```python
from build123d import *

# Parameters (mm, degrees)
SKETCH1_W            = 176
SKETCH1_H            = 90
SKETCH1_W_2          = 161
SKETCH1_H_2          = 80.5
BOSS_EXTRUDE1_DEPTH  = 5
M4_CLEARANCE_HOLE1_D = 4.5
BOSS_EXTRUDE2_DEPTH  = 90
BOSS_EXTRUDE11_DEPTH = 176
CUT_EXTRUDE1_DEPTH   = 20
BOSS_EXTRUDE12_DEPTH = 20
BOSS_EXTRUDE13_DEPTH = 5


with BuildPart() as part:
    # Sketch1 → Boss-Extrude1 (new body)
    with BuildSketch(Plane.XY):
        Rectangle(SKETCH1_W, SKETCH1_H)
        Rectangle(SKETCH1_W_2, SKETCH1_H_2, mode=Mode.SUBTRACT)
    extrude(amount=BOSS_EXTRUDE1_DEPTH)

    # M4 Clearance Hole1 (through all)
    with Locations(Plane.XY.offset(5)):
        with Locations((84, 40), (-84, -40), (-84, 40), (84, -40)):
            Hole(M4_CLEARANCE_HOLE1_D / 2)

    # Sketch7 → Boss-Extrude2 (add)
    with BuildSketch(Plane(origin=(0, 45, 0), x_dir=(1, 0, 0), z_dir=(0, 1, 0))):
        Polygon((-82.5, -5), (-88, -25.886602241), (-86, -25.886602241), (-80.5, -5), align=None)
        Polygon((80.5, -5), (60.5, -30.264322131), (62.5, -30.264322131), (82.5, -5), align=None)
    extrude(amount=-BOSS_EXTRUDE2_DEPTH)


with BuildPart() as body_2:
    # Sketch8 → Boss-Extrude11 (new body)
    with BuildSketch(Plane(origin=(88, 0, 0), x_dir=(0, 0, -1), z_dir=(1, 0, 0))):
        Polygon((-5, 40.25), (-30.264322131, 22.5), (-30.264322131, 25), (-5, 42.75), align=None)
    extrude(amount=-BOSS_EXTRUDE11_DEPTH)


with BuildPart() as body_3:
    # Mirror2: mirrored copy
    add(body_2.part.mirror(Plane.ZX))


with BuildPart() as body_2_1:
    add(body_2.part)

    # Combine2: union body 3, part
    add(body_3.part)
    add(part.part)

    # Sketch9 → Cut-Extrude1 (cut)
    with BuildSketch(Plane.XY.offset(5)):
        with BuildLine():
            Line((84, 37.75), (84, 35))
            ThreePointArc((84, 35), (86.236067977, 35.527864045), (88, 37))
            Line((88, 37), (88, 40.25))
            Line((88, 40.25), (86.236067977, 40.25))
            ThreePointArc((86.236067977, 40.25), (85.677050983, 38.5), (84, 37.75))
        make_face()
        with BuildLine():
            ThreePointArc((89, 40), (84, 45), (79, 40))
            Line((79, 40), (84, 40))
            Line((84, 40), (84, 37.75))
            ThreePointArc((84, 37.75), (85.677050983, 38.5), (86.236067977, 40.25))
            Line((86.236067977, 40.25), (88, 40.25))
            Line((88, 40.25), (88, 37))
            ThreePointArc((88, 37), (88.74341649, 38.41886117), (89, 40))
        make_face()
        with BuildLine():
            ThreePointArc((79, 40), (79.968871126, 37.041960108), (82.5, 35.230303993))
            Line((82.5, 35.230303993), (82.5, 38.322949017))
            ThreePointArc((82.5, 38.322949017), (83.197150298, 37.898112192), (84, 37.75))
            Line((84, 37.75), (84, 40))
            Line((84, 40), (79, 40))
        make_face()
        with BuildLine():
            Line((82.5, 38.322949017), (82.5, 35.230303993))
            ThreePointArc((82.5, 35.230303993), (83.241211504, 35.057911371), (84, 35))
            Line((84, 35), (84, 37.75))
            ThreePointArc((84, 37.75), (83.197150298, 37.898112192), (82.5, 38.322949017))
        make_face()
    extrude(amount=CUT_EXTRUDE1_DEPTH, mode=Mode.SUBTRACT)

    # Sketch10 → Boss-Extrude12 (add)
    with BuildSketch(Plane.XY.offset(5)):
        with BuildLine():
            Line((88, 35.527864045), (88, 37))
            ThreePointArc((88, 37), (85.531488162, 35.240321018), (82.5, 35.230303993))
            Line((82.5, 35.230303993), (82.5, 34.190524981))
            ThreePointArc((82.5, 34.190524981), (85.417610293, 34.169872981), (88, 35.527864045))
        make_face()
        with BuildLine():
            Line((82.5, 34.190524981), (82.5, 35.230303993))
            ThreePointArc((82.5, 35.230303993), (81.429126737, 35.711572472), (80.5, 36.429285786))
            ThreePointArc((80.5, 36.429285786), (79.343242015, 38.179394313), (79.006253911, 40.25))
            ThreePointArc((79.006253911, 40.25), (79.24786884, 41.554750602), (79.824176728, 42.75))
            Line((79.824176728, 42.75), (78.667317748, 42.75))
            ThreePointArc((78.667317748, 42.75), (78.523911995, 37.547968157), (82.5, 34.190524981))
        make_face()
        with BuildLine():
            ThreePointArc((79.824176728, 42.75), (80.140212612, 43.178370859), (80.5, 43.570714214))
            Line((80.5, 43.570714214), (80.5, 44.873397172))
            ThreePointArc((80.5, 44.873397172), (79.457833906, 43.920296822), (78.667317748, 42.75))
            Line((78.667317748, 42.75), (79.824176728, 42.75))
        make_face()
    extrude(amount=BOSS_EXTRUDE12_DEPTH)

    # Sketch11 → Boss-Extrude13 (add)
    with BuildSketch(Plane.XY.offset(5)):
        with BuildLine():
            Line((80.5, 35.126602828), (80.5, 40.25))
            Line((80.5, 40.25), (78.005210596, 40.25))
            ThreePointArc((78.005210596, 40.25), (78.605553216, 37.373225572), (80.5, 35.126602828))
        make_face()
    extrude(amount=-BOSS_EXTRUDE13_DEPTH)


solid = body_2_1.part
```
For this review, take the finished solid that the model builds, in its own axes (mm). A direction names the side the tool comes from. Give positions to 0.01 mm unless a question says otherwise; leave off trailing zeros. Loops run counter-clockwise (first coordinate to the right, second up) from the corner with the lowest first, then second, coordinate; pieces in that order, holes last. Notation, with made-up numbers: M 89,75.25 L 94,75.25 A20 ccw 94,103.25 Z; hole C 64.5,38 d6. An arc over 180 degrees is marked long. One line per item, written item: value. Start each with the question number.
Q1. Draft analysis for pull direction Y (two halves, no side actions). For faces 1 (the face through (0, 44, 0)), 2 (the face through (78.262, -31.779, 20.616)), 3 (the face through (72.36, -1.09, 17.81)), state which applies: released by +Y, released by -Y, zero draft, split by the parting line, or undercut.
Q2. Add section D-D (y = -33). Give the boundary of the cut face in (x, z), and give its area (3 significant figures).
Q3. Clearance check with flat-ended pins moving along their axes: pin 1 Ø1 at (x, z) = (-43, 12) entering from +Y; pin 2 Ø5 at (x, y) = (-84, 40) entering from +Z; pin 3 Ø8 at (y, z) = (-24.5, 15) entering from +X; pin 4 Ø3 at (x, y) = (-83, 40) entering from -Z. State where each tip first meets the part, or that it passes through.
Q4. Machinability: for faces 4 (the face through (-80.5, -1, 2)), 5 (the face through (81, 40, 5)), 6 (the face through (-83.9, -38.3, 17.91)), which of the approach directions +Z, -Z, +X, -X, +Y, -Y give a long, thin tool a straight path to every point of the face, cutting with its end or side? Answer none if there is none.
Q5. Add section A-A (y = -4). Give the boundary of the cut face in (x, z), and give its area (3 significant figures).
Q6. For L1, parallel to X at y = -40, z = 3; L2, parallel to Y at x = -53, z = 2.5; L3, parallel to Y at x = -34, z = 28.5, list the stretches that pass through material, from the lowest coordinate up.
Q7. Add section B-B (x = -1.5). Give the boundary of the cut face in (y, z).
Q8. Add section C-C (z = 21.5). Count the separate pieces of the cut face and the enclosed holes in it, and give its area (3 significant figures).
Reply:
1. face 1: zero draft
1. face 2: released by -Y
1. face 3: undercut
2. outline: M -88,0 L -80.5,0 L -80.5,5 L -83.22,15.32 L 72.33,15.32 L 80.5,5 L 80.5,0 L 88,0 L 88,5 L 82.5,5 L 74.33,15.32 L 88,15.32 L 88,18.88 L 71.51,18.88 L 62.5,30.26 L 60.5,30.26 L 69.51,18.88 L -84.15,18.88 L -86,25.89 L -88,25.89 L -86.15,18.88 L -88,18.88 L -88,15.32 L -85.22,15.32 L -82.5,5 L -88,5 Z
2. area: 779 mm²
3. pin 1: y = 38.18
3. pin 2: z = 25.89
3. pin 3: x = 77.75
3. pin 4: z = 0
4. face 4: -Z
4. face 5: +Z
4. face 6: +Z, -Y
5. outline: M -88,0 L -80.5,0 L -80.5,5 L -86,25.89 L -88,25.89 L -82.5,5 L -88,5 Z; M 60.5,30.26 L 80.5,5 L 80.5,0 L 88,0 L 88,5 L 82.5,5 L 62.5,30.26 Z
5. area: 167 mm²
6. L1: -88 to -86.25, -81.75 to -80.5, 80.5 to 81.75, 86.25 to 88
6. L2: -45 to -40.25, 40.25 to 45
6. L3: -26.24 to -23.74, 23.74 to 26.24
7. outline: M -45,0 L -40.25,0 L -40.25,5 L -22.5,30.26 L -25,30.26 L -42.75,5 L -45,5 Z; M 22.5,30.26 L 40.25,5 L 40.25,0 L 45,0 L 45,5 L 42.75,5 L 25,30.26 Z
8. separate pieces: 2
8. enclosed holes: 1
8. area: 1,240 mm²
